Input: part model. Units: mm. Frame: model coordinates. Face numbers are marked on the shaded views. A direction names the side the tool comes from. Give positions to 0.01 mm unless a question says otherwise; leave off trailing zeros. Loops run counter-clockwise (first coordinate to the right, second up) from the corner with the lowest first, then second, coordinate; pieces in that order, holes last. Notation, with made-up numbers: M 25.5,-15 L 73.5,-15 A33 cw 73.5,22 Z; hole C 3.25,-13.75 d9. An arc over 180 degrees is marked long. Answer as a JSON object with one key per item and string values. Group by question number.
```python
from build123d import *

# Parameters (mm, degrees)
SKETCH6_W            = 60
SKETCH6_H            = 30
SKETCH6_R            = 4
BOSS_EXTRUDE1_DEPTH  = 5
FILLET3_R            = 8
SKETCH8_W            = 18
SKETCH8_H            = 30
BOSS_EXTRUDE2_DEPTH  = 45
CUT_EXTRUDE1_DEPTH   = 20
CUT_EXTRUDE3_DEPTH   = 18
CUT_EXTRUDE4_DEPTH   = 18
BOSS_EXTRUDE4_DEPTH  = 18
SKETCH22_OUTSIDE_W   = 79.302
SKETCH22_OUTSIDE_H   = 78.983
SKETCH22_OUTSIDE_W_2 = 9
SKETCH22_OUTSIDE_H_2 = 23.546077941
CUT_EXTRUDE5_DEPTH   = 58
SKETCH26_W           = 9
SKETCH26_H           = 16.7
BOSS_EXTRUDE6_DEPTH  = 24.59
SKETCH27_R           = 3.017273599
CUT_EXTRUDE6_DEPTH   = 24.59


with BuildPart() as part:
    # Sketch6 → Boss-Extrude1 (new body)
    with BuildSketch(Plane.XY):
        Rectangle(SKETCH6_W, SKETCH6_H)
        with Locations((-20, 0)):
            Circle(SKETCH6_R, mode=Mode.SUBTRACT)
        with Locations((20, 0)):
            Circle(SKETCH6_R, mode=Mode.SUBTRACT)
    extrude(amount=BOSS_EXTRUDE1_DEPTH)

    # Fillet3
    fillet3_edges = [part.edges().sort_by_distance(p)[0] for p in [
        (30, -15, 2.5),
        (-30, -15, 2.5),
        (-30, 15, 2.5),
        (30, 15, 2.5),
    ]]
    fillet(fillet3_edges, radius=FILLET3_R)

    # Sketch8 → Boss-Extrude2 (add)
    with BuildSketch(Plane(origin=(0, 0, 0), x_dir=(-1, 0, 0), z_dir=(0, 0, -1))):
        Rectangle(SKETCH8_W, SKETCH8_H)
    extrude(amount=BOSS_EXTRUDE2_DEPTH)

    # Sketch10 → Cut-Extrude1 (cut)
    with BuildSketch(Plane.ZY.offset(9)):
        Polygon((0, 15), (-45, 2.942286341), (-45, 15), align=None)
    extrude(amount=-CUT_EXTRUDE1_DEPTH, mode=Mode.SUBTRACT)

    # Sketch17 → Cut-Extrude3 (cut)
    with BuildSketch(Plane.ZY.offset(9)):
        with BuildLine():
            Line((-19.10592487, 9.880582861), (-33.795007399, 5.944655059))
            Line((-33.795007399, 5.944655059), (-33.112800495, -15))
            Line((-33.112800495, -15), (-19.10592487, -15))
            add(Edge.make_bspline(
                [(-19.396101376, -9.592611332), (-25.746279691, -12.541160343), (-19.10592487, -15)],
                knots=[0, 0, 0, 1, 1, 1], degree=2))
            ThreePointArc((-19.396101376, -9.592611332), (-13.970550224, -2.605507152), (-19.721316162, 4.116465866))
            add(Edge.make_bspline(
                [(-19.10592487, 9.880582861), (-25.688303674, 6.38873808), (-19.721316162, 4.116465866)],
                knots=[0, 0, 0, 1, 1, 1], degree=2))
        make_face()
    extrude(amount=-CUT_EXTRUDE3_DEPTH, mode=Mode.SUBTRACT)


with BuildPart() as cut_extrude3_piece_1:
    # of the separate pieces the step leaves, piece 1, a body of its own (cut_extrude3_pieces)
    add(part.part.solids().sort_by_distance((-22, 15, 0))[0])



with BuildPart() as cut_extrude3_piece_2:
    # of the separate pieces the step leaves, piece 2, a body of its own (cut_extrude3_pieces)
    add(part.part.solids().sort_by_distance((-9, 5.944655059, -33.795007399))[0])

    # Sketch18 → Cut-Extrude4 (cut)
    with BuildSketch(Plane.ZY.offset(9)):
        Polygon((-45, 2.942286341), (-33.795007399, 5.944655059), (-33.112800495, -15), (-45, -15), align=None)
    extrude(amount=-CUT_EXTRUDE4_DEPTH, mode=Mode.SUBTRACT)


with BuildPart() as body_2:
    # Sketch20 → Boss-Extrude4 (new body)
    with BuildSketch(Plane.ZY.offset(9)):
        with BuildLine():
            Line((-37.531427351, 5.25433557), (-25.054150065, 8.387111476))
            Line((-25.054150065, 8.387111476), (-24.501921516, -16.92005289))
            Line((-24.501921516, -16.92005289), (-30.888633919, -18.84010578))
            ThreePointArc((-30.888633919, -18.84010578), (-46.53784137, -10.191639988), (-37.531427351, 5.25433557))
        make_face()
    extrude(amount=-BOSS_EXTRUDE4_DEPTH)

    # Sketch22 outside → Cut-Extrude5 (cut)
    with BuildSketch(Plane(origin=(0, -8.762066283, 2.634161307), x_dir=(1, 0, 0), z_dir=(0, -0.9576594298343689, 0.2879034846077966))):
        with Locations((0, -20.7335)):
            Rectangle(SKETCH22_OUTSIDE_W, SKETCH22_OUTSIDE_H)
        with Locations((0, -40.108877346)):
            Rectangle(SKETCH22_OUTSIDE_W_2, SKETCH22_OUTSIDE_H_2, mode=Mode.SUBTRACT)
    extrude(amount=-CUT_EXTRUDE5_DEPTH, mode=Mode.SUBTRACT)


with BuildPart() as cut_extrude3_piece_1_1:
    add(cut_extrude3_piece_1.part)

    add(body_2.part)  # Boss-Extrude6 merges body 2
    # Sketch26 → Boss-Extrude6 (add)
    with BuildSketch(Plane(origin=(0, 13.995190528, -3.75), x_dir=(1, 0, 0), z_dir=(0, 0.9659258262890699, -0.2588190451025147))):
        with Locations((0, 22.410404796)):
            Rectangle(SKETCH26_W, SKETCH26_H)
    extrude(amount=-BOSS_EXTRUDE6_DEPTH)

    # Sketch27 → Cut-Extrude6 (cut)
    with BuildSketch(Plane.ZY.offset(4.5)):
        with Locations(Location((-36.863547302, -6.273312821, 0), (0, 0, 270))):
            Circle(SKETCH27_R)
    extrude(amount=-CUT_EXTRUDE6_DEPTH, mode=Mode.SUBTRACT)


solid = cut_extrude3_piece_1_1.part
```
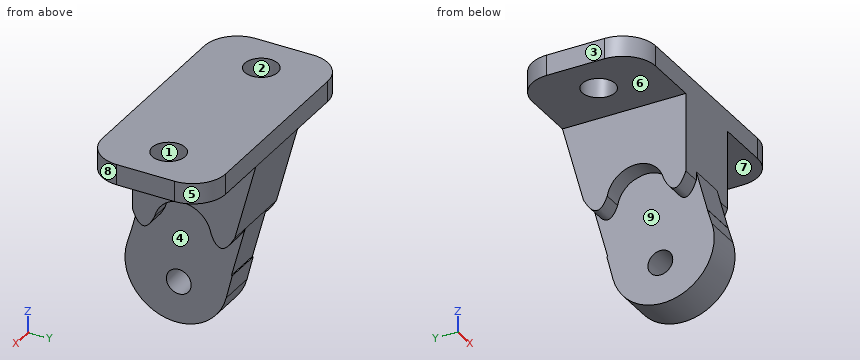
1. Mould query, pull axis X, two halves, no side actions, for the marked faces 1, 2, 3 and 4. Classes: pulls with the +X half, pulls with the -X half, needs draft (parallel to the pull), parting line crosses it, or undercut.
2. First-contact query: P1, Ø6.5, axis at x = 20, y = 0, coming from the +Z side; P2, Ø5, axis at y = -14.5, z = -1, coming from the +X side; P3, Ø14.5, axis at y = -3.5, z = -32, coming from the +X side; P4, Ø4, axis at y = 4, z = -33.5, coming from the -X side. Flat tips, straight axial feed; report the tip coordinate or a pass-through.
3. Section D-D (x = -2). Count the separate pieces of the cut face and the enclosed holes in it, then the cut area to 3 significant figures.
4. Section C-C (y = 2). Output: boundary loops of the cut face in (x, z).
5. Material intervals for L1, parallel to Y at x = 20, z = 3.25; L2, parallel to Z at x = -10.5, y = 13.5; L3, parallel to X at y = 3.5, z = -39, sorted ascending.
6. Section A-A (x = 20). Output: boundary loops of the cut face in (y, z), then the cut area to 3 significant figures.
7. Section B-B (y = -8). Output: boundary loops of the cut face in (x, z), then the cut area to 3 significant figures.
8. Reachability of the marked faces 5, 6, 7, 8 and 9 from +Z, -Z, +X, -X, +Y, -Y: full face, straight path, thin tool, end or side. Return the list, or none.
Geometry results:
{
 "1": {"face 1": "undercut", "face 2": "undercut", "face 3": "pulls with the -X half", "face 4": "pulls with the +X half"},
 "2": {"P1": "through", "P2": "x = 28.07", "P3": "x = 4.5", "P4": "x = -4.5"},
 "3": {"separate pieces": "1", "enclosed holes": "2", "area": "1,280 mm2"},
 "4": {"outline": "M -30,0 L -23.46,0 L -23.46,5 L -30,5 Z; M -16.54,0 L -9,0 L -9,-15.85 L -4.5,-15.85 L -4.5,-43.3 L 4.5,-43.3 L 4.5,-15.85 L 9,-15.85 L 9,0 L 16.54,0 L 16.54,5 L -16.54,5 Z; M 23.46,0 L 30,0 L 30,5 L 23.46,5 Z"},
 "5": {"L1": "-15 to -4, 4 to 15", "L2": "0 to 5", "L3": "-4.5 to 4.5"},
 "6": {"outline": "M -15,0 L -4,0 L -4,5 L -15,5 Z; M 4,0 L 15,0 L 15,5 L 4,5 Z", "area": "110 mm2"},
 "7": {"outline": "M -29.94,0 L -9,0 L -9,-16.31 L -4.5,-16.31 L -4.5,-34.39 L 4.5,-34.39 L 4.5,-16.31 L 9,-16.31 L 9,0 L 29.94,0 L 29.94,5 L -29.94,5 Z; M -4.5,-46.94 L 4.5,-46.94 L 4.5,-39.34 L -4.5,-39.34 Z", "area": "824 mm2"},
 "8": {"face 5": "+Z, -Z, +X, +Y", "face 6": "-Z, -X, +Y, -Y", "face 7": "-Z, +X, +Y, -Y", "face 8": "+Z, -Z, +X, -Y", "face 9": "-Z, -X"}
}
